Geometry check sheet. Reference: the model listing, model coordinates, mm. A direction names the side the tool comes from. Coordinates: 2 decimals unless noted, no trailing zeros. Loops run counter-clockwise (first coordinate to the right, second up) from the corner with the lowest first, then second, coordinate; pieces in that order, holes last. Notation, with made-up numbers: M 7.25,60.25 L 40.25,60.25 A28 ccw 40.25,81.25 Z; hole C -27.75,5.25 d5. An arc over 180 degrees is marked long. One line per question, with ' | ' between items. Start each with the question number.
from build123d import *

# Parameters (mm, degrees)
SKETCH4_R                  = 6.35
SHAFT_BORE_DEPTH           = 12.7
F_4_40_TAPPED_HOLE1_REACH  = 51.289
F_4_40_TAPPED_HOLE1_BORE_R = 1.1303
CHAMFER1_SIZE              = 0.508
CHAMFER2_SIZE              = 3.175
CHAMFER3_SIZE              = 0.508


with BuildPart() as part:
    # Sketch → Shaft (revolve)
    with BuildSketch(Plane(origin=(0, 0, 0), x_dir=(0, 0, -1), z_dir=(1, 0, 0)), mode=Mode.PRIVATE) as shaft_sk:
        Polygon((0, 0), (0, 3.175), (28.575, 3.175), (28.575, 9.525), (44.45, 9.525), (44.45, 0), align=None)
    revolve(shaft_sk.sketch.rotate(Axis((0, 0, -44.45), (0, 0, 1)), 90), axis=Axis((0, 0, -44.45), (0, 0, 1)))

    # Sketch4 → Shaft Bore (cut)
    with BuildSketch(Plane(origin=(0, 0, -44.45), x_dir=(-1, 0, 0), z_dir=(0, 0, -1))):
        Circle(SKETCH4_R)
    extrude(amount=-SHAFT_BORE_DEPTH, mode=Mode.SUBTRACT)

    # #4-40 Tapped Hole1 bore → #4-40 Tapped Hole1 (cut, up to next)
    with BuildSketch(Plane(origin=(0, -9.525, 0), x_dir=(-1, 0, 0), z_dir=(0, -1, 0)), mode=Mode.PRIVATE) as f_4_40_tapped_hole1_sk1:
        with Locations((0, 34.925)):
            Circle(F_4_40_TAPPED_HOLE1_BORE_R)
    f_4_40_tapped_hole1_tool1 = extrude(f_4_40_tapped_hole1_sk1.sketch, amount=-F_4_40_TAPPED_HOLE1_REACH, mode=Mode.PRIVATE) & part.part
    # #4-40 Tapped Hole1 bore → #4-40 Tapped Hole1 (cut, up to next)
    with BuildSketch(Plane(origin=(0, -9.525, 0), x_dir=(-1, 0, 0), z_dir=(0, -1, 0)), mode=Mode.PRIVATE) as f_4_40_tapped_hole1_sk2:
        with Locations((0, 41.275)):
            Circle(F_4_40_TAPPED_HOLE1_BORE_R)
    f_4_40_tapped_hole1_tool2 = extrude(f_4_40_tapped_hole1_sk2.sketch, amount=-F_4_40_TAPPED_HOLE1_REACH, mode=Mode.PRIVATE) & part.part
    add(f_4_40_tapped_hole1_tool1.solids().sort_by_distance((0, -9.525, -34.925))[0], mode=Mode.SUBTRACT)
    add(f_4_40_tapped_hole1_tool2.solids().sort_by_distance((0, -9.525, -41.275))[0], mode=Mode.SUBTRACT)

    # Chamfer1
    chamfer1_edges = [part.edges().sort_by_distance(p)[0] for p in [
        (3.175, 0, 0),
    ]]
    chamfer(chamfer1_edges, length=CHAMFER1_SIZE)

    # Chamfer2
    chamfer2_edges = [part.edges().sort_by_distance(p)[0] for p in [
        (3.175, 0, -28.575),
    ]]
    chamfer(chamfer2_edges, length=CHAMFER2_SIZE)

    # Chamfer3
    chamfer3_edges = [part.edges().sort_by_distance(p)[0] for p in [
        (6.35, 0, -44.45),
    ]]
    chamfer(chamfer3_edges, length=CHAMFER3_SIZE)


solid = part.part
1. Tool access check on faces 4 (the cylindrical face through (0.245, -7.908, -33.822)), 5 (the cylindrical face through (2.06, 9.3, -36.62)), 6 (the flat face through (6.2, 2, -28.575)), 7 (the cylindrical face through (1.38, -6.2, -37.93)). Record the directions out of +Z, -Z, +X, -X, +Y, -Y that give a thin tool (end or side, any length) a straight path to the whole face; none if there is none.
2. Sectioned sample at A-A (x = 0). Record the cut outline in (y, z) (3 decimals), and give its area (3 significant figures).
3. Depth check by flat-ended pin: pin 1 Ø4 at (x, z) = (-2, -9) entering from +Y (3 decimals); pin 2 Ø4 at (y, z) = (4.5, -16.5) entering from +X; pin 3 Ø6 at (x, z) = (-6, -33) entering from +Y. Enter the tip coordinate at first touch or a pass-through.
4. Sectioned sample at C-C (z = -12.5). Record the cut outline in (x, y) (3 decimals), and give its area (3 significant figures).
5. Draft check along X on faces 1 (the flat face through (-4, 6, -44.45)), 2 (the cylindrical face through (2.52, 1.93, -13.13)), 3 (the cylindrical face through (0.245, -7.908, -40.172)). Enter one of: +X half, -X half, draft (parallel to the pull), parting line (faces both ways), or undercut.
6. Sectioned sample at D-D (x = 7.5). Record the cut outline in (y, z) (3 decimals), and give its area (3 significant figures).
7. Thickness scan on line 1 (Z direction, x = 0, y = -7.35) (3 decimals); line 2 (Y direction, x = 0, z = -38.25) (3 decimals); line 3 (Z direction, x = -1.5, y = 1). Record the ranges inside material, lowest first.
8. Sectioned sample at B-B (y = 0). Record the cut outline in (x, z) (3 decimals).
Result:
1) face 4: -Y | face 5: +Z, -Z | face 6: +Z | face 7: -Z
2) outline: M -9.525,-44.45 L -6.858,-44.45 L -6.35,-43.942 L -6.35,-42.405 L -9.525,-42.405 Z; M -9.525,-40.145 L -6.35,-40.145 L -6.35,-36.055 L -9.525,-36.055 Z; M -9.525,-33.795 L -6.35,-33.795 L -6.35,-31.75 L 6.35,-31.75 L 6.35,-43.942 L 6.858,-44.45 L 9.525,-44.45 L 9.525,-28.575 L 6.35,-28.575 L 3.175,-25.4 L 3.175,-0.508 L 2.667,0 L -2.667,0 L -3.175,-0.508 L -3.175,-25.4 L -6.35,-28.575 L -9.525,-28.575 Z | area: 318 mm2
3) pin 1: stops at y = 3.175 | pin 2: stops at x = 1.96 | pin 3: stops at y = 9.04
4) outline: C 0,0 d6.35 | area: 31.7 mm2
5) face 1: draft | face 2: parting line | face 3: undercut
6) outline: M -5.872,-44.45 L 5.872,-44.45 L 5.872,-28.575 L -5.872,-28.575 Z | area: 186 mm2
7) line 1: z = -44.45 to -42.405, -40.145 to -36.055, -33.795 to -28.575 | line 2: y = -9.525 to -6.35, 6.35 to 9.525 | line 3: z = -31.75 to 0
8) outline: M -9.525,-44.45 L -6.858,-44.45 L -6.35,-43.942 L -6.35,-31.75 L 6.35,-31.75 L 6.35,-43.942 L 6.858,-44.45 L 9.525,-44.45 L 9.525,-28.575 L 6.35,-28.575 L 3.175,-25.4 L 3.175,-0.508 L 2.667,0 L -2.667,0 L -3.175,-0.508 L -3.175,-25.4 L -6.35,-28.575 L -9.525,-28.575 Z
